Part model, mm, in its own coordinate system. Round coordinates to 2 decimals unless told otherwise and drop trailing zeros. Order: outer loops, then holes, each group sorted by start corner. A loop starts at its lowest first (then second) coordinate and runs counter-clockwise, first axis right, second up. Notation, with made-up numbers: (26, -30.75) - (83, -30.75) arc R30 cw to (83, 3.25) - close; hole circle Ø6 at (15, 6). An arc over 180 degrees is marked (long way). Answer as a JSON object with one key per item and string values.
```python
from build123d import *

# Parameters (mm, degrees)
EXTRUDE_1_DEPTH     = 400
SKETCH_2_R          = 1.7
CUT_EXTRUDE_1_DEPTH = 5
SKETCH_3_R          = 1.7
CUT_EXTRUDE_2_DEPTH = 5


with BuildPart() as part:
    # Эскиз1 → Вытянуть1 (new body)
    with BuildSketch(Plane.XY):
        with BuildLine():
            Line((0, 0), (2, 0))
            Line((2, 0), (2, 7))
            ThreePointArc((2, 7), (2.292893219, 7.707106781), (3, 8))
            Line((3, 8), (10, 8))
            Line((10, 8), (10, 10))
            Line((10, 10), (2, 10))
            ThreePointArc((2, 10), (0.585786438, 9.414213562), (0, 8))
            Line((0, 8), (0, 0))
        make_face()
    extrude(amount=EXTRUDE_1_DEPTH)

    # Эскиз2 → Вырез-Вытянуть1 (cut)
    with BuildSketch(Plane(origin=(0, 10, 0), x_dir=(-1, 0, 0), z_dir=(0, 1, 0))):
        with Locations(Location((-4, 396, 0), (0, 0, 90))):
            Circle(SKETCH_2_R)
        with Locations(Location((-4, 4, 0), (0, 0, 53.968120928))):
            Circle(SKETCH_2_R)
        with Locations(Location((-4, 204, 0), (0, 0, 53.968120928))):
            Circle(SKETCH_2_R)
        with Locations(Location((-4, 196, 0), (0, 0, 90))):
            Circle(SKETCH_2_R)
    extrude(amount=-CUT_EXTRUDE_1_DEPTH, mode=Mode.SUBTRACT)

    # Эскиз3 → Вырез-Вытянуть2 (cut)
    with BuildSketch(Plane.ZY):
        with Locations((388, 4)):
            Circle(SKETCH_3_R)
        with Locations((380, 4)):
            Circle(SKETCH_3_R)
        with Locations((20, 4)):
            Circle(SKETCH_3_R)
        with Locations((12, 4)):
            Circle(SKETCH_3_R)
    extrude(amount=-CUT_EXTRUDE_2_DEPTH, mode=Mode.SUBTRACT)


solid = part.part
```
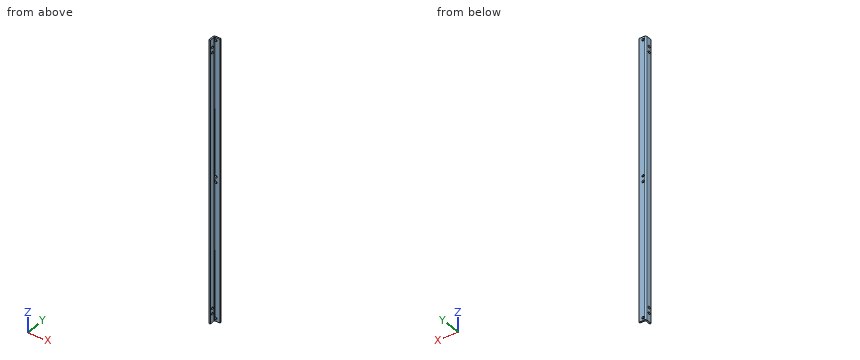
Item 1: Probe L1, parallel to Z at x = 4, y = 9; L2, parallel to X at y = 8.5, z = 4; L3, parallel to Y at x = 5.25, z = 305.5. List the from-to ranges inside material, lowest first. Write a range as from..to.
Taken from the geometry:
{"L1": "0..2.3, 5.7..194.3, 197.7..202.3, 205.7..394.3, 397.7..400", "L2": "0.06..2.3, 5.7..10", "L3": "8..10"}
Item 2: Drop flat-ended pins along their axis: P1, Ø5.5, axis at x = 4, z = 204, coming from the +Y side; P2, Ø1, axis at x = 9, z = 300, coming from the -Y side. Give the stop position or say it passes through.
Taken from the geometry:
{"P1": "y = 10", "P2": "y = 8"}
Item 3: Cut at B-B (z = 98.5). Write the cut outline in (x, y), plus the area to 3 significant figures.
Taken from the geometry:
{"outline": "(0, 0) - (2, 0) - (2, 7) arc R1 cw to (3, 8) - (10, 8) - (10, 10) - (2, 10) arc R2 ccw to (0, 8) - close", "area": "35.4 mm2"}
Item 4: Cut at A-A (y = 4). Write the cut outline in (x, z).
Taken from the geometry:
{"outline": "(0, 0) - (2, 0) - (2, 10.3) - (0, 10.3) - close; (0, 13.7) - (2, 13.7) - (2, 18.3) - (0, 18.3) - close; (0, 21.7) - (2, 21.7) - (2, 378.3) - (0, 378.3) - close; (0, 381.7) - (2, 381.7) - (2, 386.3) - (0, 386.3) - close; (0, 389.7) - (2, 389.7) - (2, 400) - (0, 400) - close"}
